Can you work these out from the model? Positions are in its coordinate system, mm. A direction names the side the tool comes from. Give positions to 0.01 mm unless a question says otherwise; leave off trailing zeros. Order: outer loops, then holes, each group sorted by start corner. A loop starts at its lowest first (then second) coordinate and runs counter-clockwise, first axis right, second up. Notation, with made-up numbers: (6, 30.25) -> (50, 30.25) arc R23 cw to (50, 43.25) -> close; hole circle Ø7 at (78, 1.25). An arc over 180 degrees is marked (long way). Answer as a JSON object with one key per item and string values.
Autodesk Inventor part; units mm, degrees
ref_plane "YZ Plane" through (0, 0, 0) normal (1, 0, 0) x (0, 1, 0)
ref_plane "XZ Plane" through (0, 0, 0) normal (0, 1, 0) x (-1, 0, 0)
ref_plane "XY Plane" through (0, 0, 0) normal (0, 0, 1) x (1, 0, 0)
sketch "Sketch1" plane through (0, 0, 0) normal (0, 0, 1) x (1, 0, 0)
  line L0 (-13.202, 13.202) -> (12.198, 13.202)
  line L1 (12.198, 13.202) -> (12.198, -12.198)
  line L2 (12.198, -12.198) -> (-13.202, -12.198)
  line L3 (-13.202, -12.198) -> (-13.202, 13.202)
  point P0 (0, 0)
  dimension "d0" = 25.4
  dimension "d1" = 25.4
extrude "Extrusion1" add sketch "Sketch1" along normal blind 101.6
sketch "Sketch6" plane through (12.198, 13.202, 101.6) normal (1, 0, 0) x (0, 0, -1)
  line L0 (101.6, 0) -> (101.6, -25.4)
  line L1 (101.6, -25.4) -> (0, -25.4)
  line L2 (101.6, 0) -> (101.6, -25.4)
  line L3 (101.6, 0) -> (0, 0)
  line L4 (0, -25.4) -> (0, 0)
  line L5 (0, -25.4) -> (0, 0)
  point P0 (101.6, -13.202)
  point P1 (88.9, -6.35)
  point P2 (88.9, -19.05)
  point P3 (101.6, -19.05)
  point P4 (101.6, -6.35)
  point P5 (12.7, -6.35)
  point P6 (12.7, -19.05)
  point P7 (0, -19.05)
  point P8 (0, -6.35)
  dimension "d51" = 12.7
  dimension "d52" = 6.35
  dimension "d53" = 12.7
  dimension "d54" = 6.35
  dimension "d55" = 12.7
  dimension "d56" = 6.35
  dimension "d57" = 12.7
  dimension "d58" = 6.35
sketch "Sketch7" plane through (12.198, 13.202, 101.6) normal (1, 0, 0) x (0, 0, -1)
  line L0 (0, -25.4) -> (0, 0)
  line L1 (101.6, 0) -> (0, 0)
  point P0 (101.6, -13.202)
  point P1 (25.4, -6.35)
  point P2 (25.4, -19.05)
  point P3 (76.2, -6.35)
  point P4 (76.2, -19.05)
  point P5 (0, -6.35)
  dimension "d66" = 0
  dimension "d67" = 0
  dimension "d68" = 0
  dimension "d69" = 0
  dimension "d70" = 25.4
  dimension "d71" = 6.35
  dimension "d72" = 19.05
  dimension "d73" = 76.2
hole "Hole3" at (12.198, 6.852, 76.2) at (12.198, -5.848, 76.2) at (12.198, 6.852, 25.4) at (12.198, -5.848, 25.4) direction (-1, 0, 0) diameter 3.175 depth 25.4 tip angle 118.188
sketch "Sketch8" plane through (0, 0, 101.6) normal (0, 0, 1) x (1, 0, 0)
  line L0 (-13.202, 13.202) -> (-13.202, -12.198)
  line L1 (-13.202, -12.198) -> (12.198, -12.198)
  point P0 (0, 0)
  point P1 (-8.122, 0.502)
  point P2 (-0.502, 0.502)
  point P3 (7.118, 0.502)
  dimension "d81" = 0
  dimension "d82" = 5.08
  dimension "d83" = 12.7
  dimension "d84" = 12.7
  dimension "d85" = 0
  dimension "d86" = 20.32
hole "Hole4" at (-8.122, 0.502, 101.6) at (-0.502, 0.502, 101.6) at (7.118, 0.502, 101.6) direction (0, 0, -1) diameter 6.477 end through all
hole "Hole5" at (12.198, 6.852, 12.7) at (12.198, -5.848, 12.7) at (12.198, 6.852, 88.9) at (12.198, -5.848, 88.9) direction (-1, 0, 0) diameter 4.318 end through all counterbore diameter 7.62 counterbore depth 4.318
properties part number "BottomOfBackElevatorFrame"
1. If we section it at A-A on x = -6.5: Count the separate pieces of the cut face and the enclosed holes in it, then the cut area to 3 significant figures.
Worked answers:
{"separate pieces": "2", "enclosed holes": "8", "area": "1,920 mm²"}
2. If we section it at D-D on z = 76.2: Please give me the cut outline in (x, y), then the cut area to 3 significant figures.
Worked answers:
{"outline": "(-13.2, -12.2) -> (12.2, -12.2) -> (12.2, -7.44) -> (-13.2, -7.44) -> close; (-13.2, -4.26) -> (12.2, -4.26) -> (12.2, 5.26) -> (-13.2, 5.26) -> close; (-13.2, 8.44) -> (12.2, 8.44) -> (12.2, 13.2) -> (-13.2, 13.2) -> close; hole circle Ø6.48 at (-8.12, 0.5); hole circle Ø6.48 at (-0.5, 0.5); hole circle Ø6.48 at (7.12, 0.5)", "area": "385 mm²"}
3. Please list where these lines run through material, in increasing order: L1, parallel to Z at x = -2.25, y = 5.75; L2, parallel to Z at x = 8.5, y = -5; L3, parallel to Y at x = 5.75, z = 76.2.
Worked answers:
{"L1": "0 to 10.84, 14.56 to 24.26, 26.54 to 75.06, 77.34 to 87.04, 90.76 to 101.6", "L2": "0 to 8.99, 16.41 to 24.06, 26.74 to 74.86, 77.54 to 85.19, 92.61 to 101.6", "L3": "-12.2 to -7.44, -4.26 to -2.43, 3.44 to 5.26, 8.44 to 13.2"}
4. Will these pins go through, and if not, where does the flat tip stop? pin 1 Ø4 at (x, y) = (-0.502, 0.502) entering from +Z; pin 2 Ø6 at (y, z) = (-5.848, 12.7) entering from +X.
Worked answers:
{"pin 1": "through", "pin 2": "x = 7.88"}
5. If we section it at B-B on z = 12.7: Please give me the cut outline in (x, y).
Worked answers:
{"outline": "(-13.2, -12.2) -> (12.2, -12.2) -> (12.2, -9.66) -> (7.88, -9.66) -> (7.88, -8.01) -> (-13.2, -8.01) -> close; (-13.2, -3.69) -> (7.88, -3.69) -> (7.88, -2.65) arc R3.24 cw (long way) to (7.88, 3.65) -> (7.88, 4.69) -> (-13.2, 4.69) -> close; (-13.2, 9.01) -> (7.88, 9.01) -> (7.88, 10.66) -> (12.2, 10.66) -> (12.2, 13.2) -> (-13.2, 13.2) -> close; (9.13, -2.04) -> (12.2, -2.04) -> (12.2, 3.04) -> (9.13, 3.04) arc R3.24 cw to start; hole circle Ø6.48 at (-8.12, 0.5); hole circle Ø6.48 at (-0.5, 0.5)"}
6. If we mould it in two halves opening along Y, with no side actions, what happens to faces 3 (the face through (2, 4, 0)), 4 (the face through (-2.809, -3.933, 87.904)), 5 (the face through (-1, 13.202, 50)), 6 (the face through (0, -12.198, 50))? For each: +Y half, -Y half, draft (parallel to the pull), parting line (faces both ways), or undercut.
Worked answers:
{"face 3": "draft", "face 4": "undercut", "face 5": "+Y half", "face 6": "-Y half"}
7. For faces 1 (the face through (9.991, -0.992, 50.089)), 2 (the face through (10.009, -9.626, 13.196)), which set-ups out of +Z, -Z, +X, -X, +Y, -Y let a thin tool reach every point of the face, with its end or its side?
Worked answers:
{"face 1": "+Z, -Z", "face 2": "+X"}
8. If we section it at C-C on y = 1.5: Please give me the cut outline in (x, z), then the cut area to 3 significant figures.
Worked answers:
{"outline": "(-13.2, 0) -> (-11.2, 0) -> (-11.2, 101.6) -> (-13.2, 101.6) -> close; (-5.04, 0) -> (-3.58, 0) -> (-3.58, 101.6) -> (-5.04, 101.6) -> close; (2.58, 0) -> (4.04, 0) -> (4.04, 101.6) -> (2.58, 101.6) -> close; (10.2, 0) -> (12.2, 0) -> (12.2, 101.6) -> (10.2, 101.6) -> close", "area": "703 mm²"}
